Part print with two shaded views. Sizes in mm from the minimum x, y, z corner. A direction names the side the tool comes from. Coordinates: 2 decimals unless noted, no trailing zeros.
(1) Wall check: L1, parallel to Z at x = 19.05, y = 16.5 (1 decimal); L2, parallel to Y at x = 45, z = 41; L3, parallel to X at y = 1.5, z = 60.5. Give the ranges that are in metal, low to high.
(2) Flat gauge pins, fed straight in: P1, Ø15, axis at x = 19.05, z = 44.45, coming from the +Y side; P2, Ø5, axis at x = 44.45, z = 19.05, coming from the +Y side; P3, Ø10, axis at x = 30, y = 10.5, coming from the +Z side; P4, Ø14.5, axis at x = 59, z = 69, coming from the -Y side. Where does each tip first touch, or does it go through?
(3) Tool access for the marked faces 1, 2, 3, 4 and 5: list every direction of +Z, -Z, +X, -X, +Y, -Y with a clear straight run to the whole face (end or side of a thin tool).
(4) Slice it at B-B (y = 11.25). Give the number of separate pieces and of enclosed holes in the cut face, and give its area (3 significant figures).
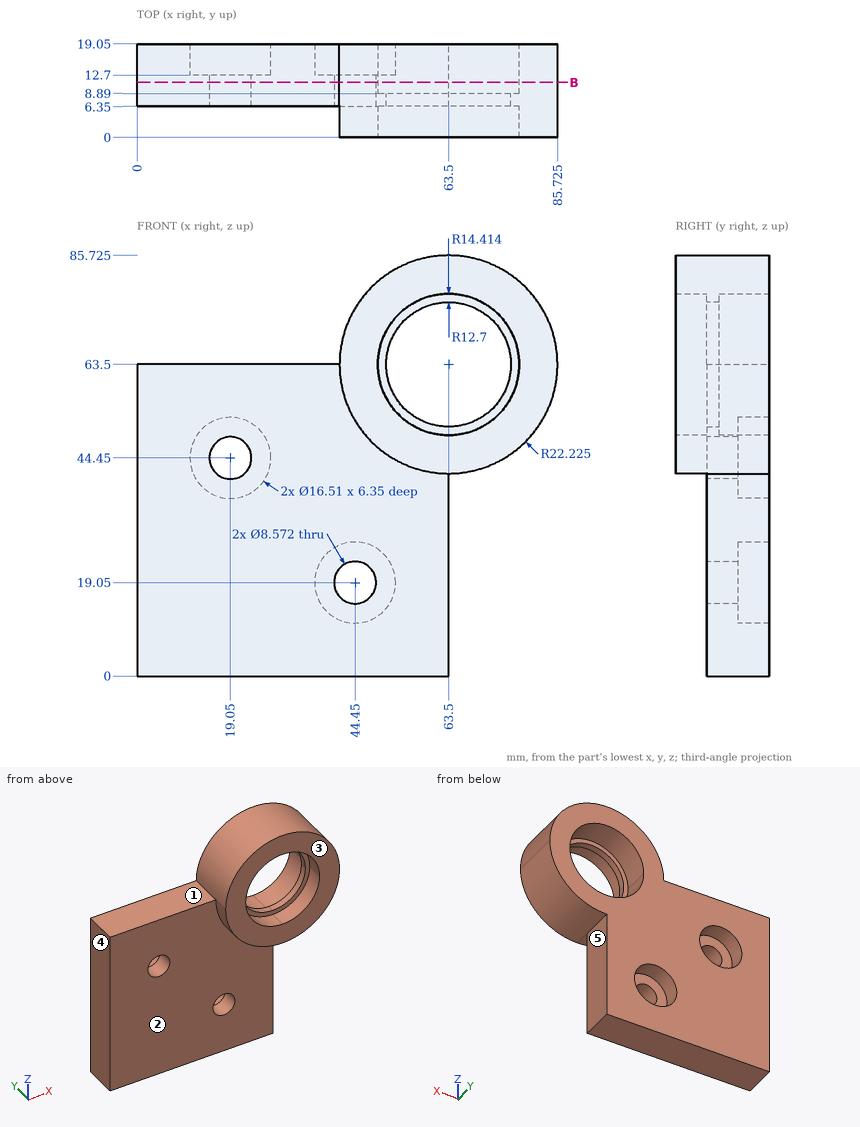
Response values:
1. L1: z = 0 to 36.2, 52.7 to 63.5
1. L2: y = 6.35 to 19.05
1. L3: x = 41.48 to 49.4, 77.6 to 85.52
2. P1: stops at y = 12.7
2. P2: passes through
2. P3: stops at z = 63.5
2. P4: stops at y = 6.35
3. face 1: +Z, -X, +Y, -Y
3. face 2: -Z, -X, -Y
3. face 3: +Z, -Z, +X, -X, -Y
3. face 4: +Z, -Z, -X, +Y, -Y
3. face 5: -Z, +X, +Y, -Y
4. separate pieces: 1
4. enclosed holes: 3
4. area: 4,430 mm2
